Verification items for the finished model (mm, model axes). Coordinates: 2 decimals unless noted, no trailing zeros. Write each loop counter-clockwise with the first axis right and the second up, starting at its lowest first coordinate (ties: lowest second). Pieces come first, ordered by that corner, then holes. Notation, with made-up numbers: (68.25, -5.5) -> (119.25, -5.5) arc R27 cw to (119.25, 27.5) -> close; hole circle Ø1 at (65, 77). An arc over 180 degrees is marked (long way). Write each question's results on one line, items separated by ' | '. Start each with the question number.
from build123d import *

# Parameters (mm, degrees)
F1_DEPTH = 991.5
F2_W     = 820
F2_H     = 26
F3_DEPTH = 13
F4_R     = 10
F5_DEPTH = 40


with BuildPart() as f1:
    # F0 (on Top) → F1 (new body, symmetric)
    with BuildSketch(Plane.XY):
        Polygon((-423, -6), (-423, -20), (423, -20), (423, -6), (410, -6), (410, 20), (-410, 20), (-410, -6), align=None)
    extrude(amount=F1_DEPTH, both=True)

    # F2 (on face) → F3 (cut)
    with BuildSketch(Plane.XY.offset(991.5)):
        with Locations((0, 7)):
            Rectangle(F2_W, F2_H)
    extrude(amount=-F3_DEPTH, mode=Mode.SUBTRACT)

    # F4 (on face) → F5 (cut, through all)
    with BuildSketch(Plane(origin=(0, 20, 0), x_dir=(-1, 0, 0), z_dir=(0, 1, 0))):
        with Locations((-360, 58.5)):
            Circle(F4_R)
        with Locations((-360, -13.5)):
            Circle(F4_R)
    extrude(amount=-F5_DEPTH, mode=Mode.SUBTRACT)


solid = f1.part
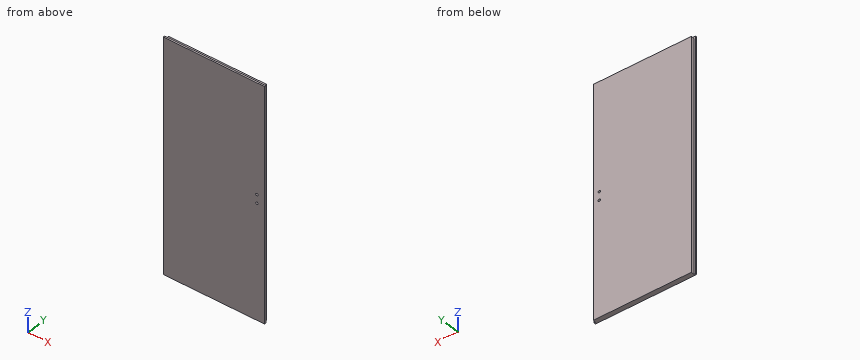
1. Depth check by flat-ended pin: pin 1 Ø16 at (x, z) = (360, -13.5) entering from +Y; pin 2 Ø13 at (y, z) = (3, -220) entering from -X; pin 3 Ø8 at (y, z) = (7, -456.5) entering from +X; pin 4 Ø6 at (y, z) = (-3.5, -289.5) entering from -X. Enter the tip coordinate at first touch or a pass-through.
2. Material ranges on probe 1 along Z at (x, y) = (360, 12.5); probe 2 along Z at (x, y) = (360, -9); probe 3 along X at (y, z) = (-15, -11.5), recorded low to high. Write a range as from..to.
3. Sectioned sample at B-B on y = 6. Record the cut outline in (x, z), plus the area to 3 significant figures.
4. Sectioned sample at A-A on z = 345. Record the cut outline in (x, y).
Computed values:
1) pin 1: passes through | pin 2: stops at x = -410 | pin 3: stops at x = 410 | pin 4: stops at x = -423
2) probe 1: z = -991.5..-23.5, -3.5..48.5, 68.5..978.5 | probe 2: z = -991.5..-23.5, -3.5..48.5, 68.5..991.5 | probe 3: x = -423..350.2, 369.8..423
3) outline: (-410, -991.5) -> (410, -991.5) -> (410, 978.5) -> (-410, 978.5) -> close; hole circle Ø20 at (360, -13.5); hole circle Ø20 at (360, 58.5) | area: 1,610,000 mm^2
4) outline: (-423, -20) -> (423, -20) -> (423, -6) -> (410, -6) -> (410, 20) -> (-410, 20) -> (-410, -6) -> (-423, -6) -> close
